```python
from build123d import *

# Parameters (mm, degrees)
F2_SIZE = 2


with BuildPart() as f1:
    # F0 (on Front) → F1 (revolve)
    with BuildSketch(Plane.XZ):
        with BuildLine():
            Line((19.120241, 50.317076), (0, 50))
            Line((0, 50), (0, 0))
            Line((0, 0), (45, 0))
            Line((45, 0), (45, 15.742122))
            ThreePointArc((45, 15.742122), (43.535534, 19.277656), (40, 20.742122))
            Line((40, 20.742122), (38.317099, 20.742122))
            ThreePointArc((38.317099, 20.742122), (35.552971, 21.575637), (33.71042, 23.798285))
            Line((33.71042, 23.798285), (23.809825, 47.2616))
            ThreePointArc((23.809825, 47.2616), (21.932636, 49.507021), (19.120241, 50.317076))
        make_face()
    revolve(axis=Axis((0, 0, 15.365856), (0, 0, -1)))

    # F2
    f2_edges = [f1.edges().sort_by_distance(p)[0] for p in [
        (-45, 0, 0),
    ]]
    chamfer(f2_edges, length=F2_SIZE)


solid = f1.part
```
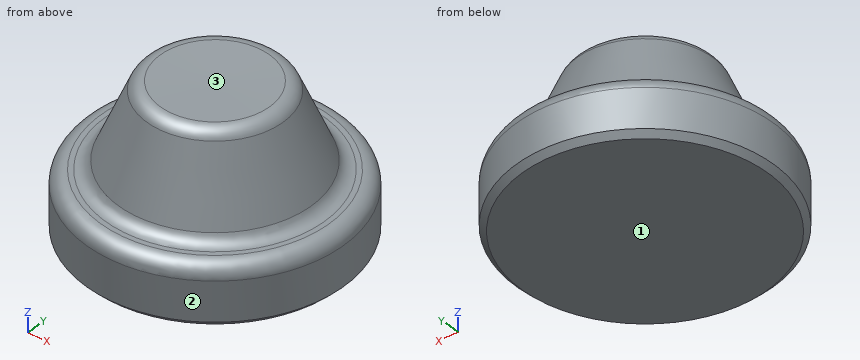
For this review, take the finished solid that the model builds, in its own axes (mm). Face numbers are marked on the shaded views. Coordinates: 2 decimals unless noted, no trailing zeros. Write each loop counter-clockwise with the first axis right and the second up, starting at its lowest first coordinate (ties: lowest second). Pieces come first, ordered by that corner, then holes. Notation, with made-up numbers: (44.25, 7.5) -> (85.25, 7.5) arc R17 cw to (85.25, 40.5) -> close; hole circle Ø11 at (-3.5, 77). An arc over 180 degrees is marked (long way). Put each result on its own line as item: value.
Q1. Clearance check with flat-ended pins moving along their axes: pin 1 Ø1 at (x, z) = (12, 44) entering from -Y; pin 2 Ø10 at (y, z) = (8, 24.5) entering from +X; pin 3 Ø1.5 at (x, y) = (11.5, -33) entering from +Z. State where each tip first meets the part, or that it passes through.
From the geometry:
pin 1: stops at y = -22.5
pin 2: stops at x = 42.62
pin 3: stops at z = 22.91
Q2. Take a section at A-A, the plane z = 5.5. State the section outline as (x, y) points.
From the geometry:
outline: circle Ø90 at (0, 0)
Q3. The part is to be moulded in two halves that separate along X. For the marked faces 1, 2 and 3, say which applies: +X half, -X half, draft (parallel to the pull), parting line (faces both ways), or undercut.
From the geometry:
face 1: draft
face 2: parting line
face 3: undercut
Q4. Take a section at B-B, the plane z = 36. State the section outline as (x, y) points.
From the geometry:
outline: circle Ø57.12 at (0, 0)
Q5. Wall thickness on L1, parallel to Y at x = -1, z = 10.5; L2, parallel to Y at x = 24, z = 22; L3, parallel to Z at x = -29, y = 19: over which ranges is each line inside the solid? List them lowest first.
From the geometry:
L1: y = -44.99 to 44.99
L2: y = -25.48 to 25.48
L3: z = 0 to 22.32
